```python
from build123d import *

# Parameters (mm, degrees)
SKETCH1_R           = 16.5
BOSS_EXTRUDE1_DEPTH = 50
SKETCH4_W           = 115
SKETCH4_H           = 30
BOSS_EXTRUDE2_DEPTH = 105
FILLET1_R           = 20
FILLET2_R           = 20
FILLET3_R           = 20
FILLET4_R           = 20
FILLET5_R           = 5
CUT_EXTRUDE2_DEPTH  = 138
BOSS_EXTRUDE4_DEPTH = 8


with BuildPart() as part:
    # Sketch1 → Boss-Extrude1 (new body, symmetric)
    with BuildSketch(Plane.XY):
        with BuildLine():
            Line((40, -107.819293264), (40, 0))
            Line((40, 0), (-40, 0))
            Line((-40, 0), (-40, -107.819293264))
            ThreePointArc((-40, -107.819293264), (-35.036523196, -109.532835453), (-30, -111.018016556))
            Line((-30, -111.018016556), (-30, -165))
            Line((-30, -165), (30, -165))
            Line((30, -165), (30, -111.018016556))
            ThreePointArc((30, -111.018016556), (35.036523196, -109.532835453), (40, -107.819293264))
        make_face()
        with Locations((0, -75)):
            Circle(SKETCH1_R, mode=Mode.SUBTRACT)
        with BuildLine():
            Line((-40, 0), (40, 0))
            Line((40, 0), (40, 107.819293264))
            ThreePointArc((40, 107.819293264), (0, 115), (-40, 107.819293264))
            Line((-40, 107.819293264), (-40, 0))
        make_face()
        with Locations((0, 75)):
            Circle(SKETCH1_R, mode=Mode.SUBTRACT)
    extrude(amount=BOSS_EXTRUDE1_DEPTH, both=True)

    # Sketch4 → Boss-Extrude2 (add, symmetric)
    with BuildSketch(Plane.XY):
        with Locations((0, -180)):
            Rectangle(SKETCH4_W, SKETCH4_H)
    extrude(amount=BOSS_EXTRUDE2_DEPTH, both=True)

    # Fillet1
    fillet1_edges = [part.edges().sort_by_distance(p)[0] for p in [
        (-30, -165, 0),
    ]]
    fillet(fillet1_edges, radius=FILLET1_R)

    # Fillet2
    fillet2_edges = [part.edges().sort_by_distance(p)[0] for p in [
        (0, -165, 50),
    ]]
    fillet(fillet2_edges, radius=FILLET2_R)

    # Fillet3
    fillet3_edges = [part.edges().sort_by_distance(p)[0] for p in [
        (0, -165, -50),
    ]]
    fillet(fillet3_edges, radius=FILLET3_R)

    # Fillet4
    fillet4_edges = [part.edges().sort_by_distance(p)[0] for p in [
        (30, -165, 0),
    ]]
    fillet(fillet4_edges, radius=FILLET4_R)

    # Fillet5
    fillet5_edges = [part.edges().sort_by_distance(p)[0] for p in [
        (-30, -111.018016556, 0),
        (30, -111.018016556, 0),
    ]]
    fillet(fillet5_edges, radius=FILLET5_R)

    # Sketch6 → Cut-Extrude2 (cut)
    with BuildSketch(Plane.ZY.offset(40)):
        with BuildLine():
            Line((0, 40), (-50, 40))
            Line((-50, 40), (-50, -40))
            Line((-50, -40), (0, -40))
            ThreePointArc((0, -40), (40, 0), (0, 40))
        make_face()
    extrude(amount=-CUT_EXTRUDE2_DEPTH, mode=Mode.SUBTRACT)

    # Sketch8 → Boss-Extrude4 (add)
    with BuildSketch(Plane.XY.offset(50)):
        Polygon((-39.81738938, -22.5), (-40, 22.5), (40, 22.5), (39.81738938, -22.5), align=None)
    extrude(amount=BOSS_EXTRUDE4_DEPTH)


solid = part.part
```
The listing builds one solid part. Answer for the finished solid, in the listing's coordinates (mm). A direction names the side the tool comes from. Coordinates: 2 decimals unless noted, no trailing zeros. Loops run counter-clockwise (first coordinate to the right, second up) from the corner with the lowest first, then second, coordinate; pieces in that order, holes last. Notation, with made-up numbers: (77.5, 41) -> (87.5, 41) arc R8 ccw to (87.5, 50) -> close; hole circle Ø6 at (84.25, 57). An arc over 180 degrees is marked (long way). Return JSON: item names as keys, results as strings. Group by question number.
(1) A cutting plane is placed at C-C on y = 0. Write down the section's boundary in (x, z).
(2) Determine the mould class of faces 1 (the flat face through (-30, -130, 1)), 2 (the flat face through (-1, -180, -105)), 3 (the cylindrical face through (0.7, -161.5, -58.7)) for opening direction Y: released by +Y, released by -Y, zero draft, split by the parting line, or undercut.
(3) A cutting plane is placed at A-A on y = -75. Write down the section's boundary in (x, z).
(4) Given pin 1 Ø3 at (x, y) = (-5, -138) entering from -Z; pin 2 Ø12 at (x, z) = (-42.5, -56) entering from +Y; pin 3 Ø4 at (x, z) = (-17.5, 52.5) entering from +Y, each flat-ended and moving along its own axis, determine where each tip first touches the part or whether it passes through.
(5) Find the intervals of material crossed by probe 1 along Y at (x, z) = (0, -0.5); probe 2 along Y at (x, z) = (-32, -6); probe 3 along Y at (x, z) = (-36, 14), in increasing order. Write a range as from..to.
(6) A cutting plane is placed at D-D on z = -83.5. Write down the section's boundary in (x, y).
(7) A cutting plane is placed at B-B on x = 0. Write down the section's boundary in (y, z).
(8) Which of the six approach directions +Z, -Z, +X, -X, +Y, -Y give full straight-line access (tool end or side, diameter ignored) to faces 4 (the cylindrical face through (36.014, -159.297, 0.98)), 5 (the flat face through (1, -22.5, 54)), 6 (the flat face through (-1, 95, -50)), 7 (the flat face through (-1, 22.5, 54))?
The answers:
{
 "1": {"outline": "(-40, 40) -> (40, 40) -> (40, 50) -> (39.91, 50) -> (39.91, 58) -> (-39.91, 58) -> (-39.91, 50) -> (-40, 50) -> close"},
 "2": {"face 1": "undercut", "face 2": "zero draft", "face 3": "released by +Y"},
 "3": {"outline": "(-40, -50) -> (-16.5, -50) -> (-16.5, 50) -> (-40, 50) -> close; (16.5, -50) -> (40, -50) -> (40, 50) -> (16.5, 50) -> close"},
 "4": {"pin 1": "stops at z = -50", "pin 2": "stops at y = -159.76", "pin 3": "stops at y = 22.5"},
 "5": {"probe 1": "y = -195..-91.5, -58.5..-40, 40..58.5, 91.5..115", "probe 2": "y = -195..-153.72, -110.78..-40, 40..110.46", "probe 3": "y = -195..-159.28, -109.22..-37.47, 37.47..109.22"},
 "6": {"outline": "(-57.5, -195) -> (57.5, -195) -> (57.5, -165) -> (-57.5, -165) -> close"},
 "7": {"outline": "(-195, -105) -> (-165, -105) -> (-165, -70) arc R20 cw to (-145, -50) -> (-91.5, -50) -> (-91.5, 50) -> (-145, 50) arc R20 cw to (-165, 70) -> (-165, 105) -> (-195, 105) -> close; (-58.5, -50) -> (-40, -50) -> (-40, 0) arc R40 cw to (40, 0) -> (40, -50) -> (58.5, -50) -> (58.5, 50) -> (22.5, 50) -> (22.5, 58) -> (-22.5, 58) -> (-22.5, 50) -> (-58.5, 50) -> close; (91.5, -50) -> (115, -50) -> (115, 50) -> (91.5, 50) -> close"},
 "8": {"face 4": "+Z, -Z, +X", "face 5": "+Z, +X, -X", "face 6": "-Z, +X, -X, +Y", "face 7": "+Z, +X, -X, +Y"}
}
